Check sheet for the modelled part. Datum: model origin and axes. Units: mm. Face numbers are marked on the shaded views. Coordinates: 2 decimals unless noted, no trailing zeros. Loops run counter-clockwise (first coordinate to the right, second up) from the corner with the lowest first, then second, coordinate; pieces in that order, holes last. Notation, with made-up numbers: (54, 77) -> (111, 77) arc R26 cw to (111, 101) -> close; hole circle Ø7 at (-3.5, 83.25). An arc over 180 degrees is marked (long way). Use CSV: the item, a comma, the result in double quotes.
```python
from build123d import *

# Parameters (mm, degrees)
CROQUIS1_R              = 22.05
CROQUIS1_R_2            = 20.05
SALIENTE_EXTRUIR1_DEPTH = 16
CROQUIS1_4_R            = 17.95
CROQUIS1_4_R_2          = 16.2
SALIENTE_EXTRUIR2_DEPTH = 12.5
SALIENTE_EXTRUIR4_START = -5
CROQUIS1_6_R            = 22.05
CROQUIS1_6_R_2          = 20.05
CROQUIS1_6_R_3          = 17.95
CROQUIS1_6_R_4          = 16.2
SALIENTE_EXTRUIR4_DEPTH = 5
CORTAR_EXTRUIR1_REACH   = 39.595
CROQUIS4_R              = 11.05
CROQUIS4_R_2            = 1.25
CROQUIS5_R              = 2.5
CROQUIS5_R_2            = 1.25
CORTAR_EXTRUIR2_DEPTH   = 3
REDONDEO1_R             = 1
REDONDEO3_R             = 1
REDONDEO4_R             = 1


with BuildPart() as part:
    # Croquis1 → Saliente-Extruir1 (new body)
    with BuildSketch(Plane(origin=(0, 0, 0), x_dir=(1, 0, 0), z_dir=(0, 1, 0))):
        with Locations(Location((0, 0, 0), (0, 0, 270))):
            Circle(CROQUIS1_R)
        with Locations(Location((0, 0, 0), (0, 0, 270))):
            Circle(CROQUIS1_R_2, mode=Mode.SUBTRACT)
    extrude(amount=SALIENTE_EXTRUIR1_DEPTH)



with BuildPart() as body_2:
    # Croquis1_4 → Saliente-Extruir2 (new body)
    with BuildSketch(Plane(origin=(0, 0, 0), x_dir=(1, 0, 0), z_dir=(0, 1, 0))):
        with Locations(Location((0, 0, 0), (0, 0, 270))):
            Circle(CROQUIS1_4_R)
        with Locations(Location((0, 0, 0), (0, 0, 270))):
            Circle(CROQUIS1_4_R_2, mode=Mode.SUBTRACT)
    extrude(amount=SALIENTE_EXTRUIR2_DEPTH)


with BuildPart() as part_1:
    add(part.part)

    add(body_2.part)  # Saliente-Extruir4 merges body 2
    # Croquis1_6 → Saliente-Extruir4 (add)
    # profile 1 of 4: a face of its own
    with BuildSketch(Plane(origin=(0, 0, 0), x_dir=(1, 0, 0), z_dir=(0, 1, 0)).offset(SALIENTE_EXTRUIR4_START)):
        with Locations(Location((0, 0, 0), (0, 0, 270))):
            Circle(CROQUIS1_6_R)
        with Locations(Location((0, 0, 0), (0, 0, 270))):
            Circle(CROQUIS1_6_R_2, mode=Mode.SUBTRACT)
    # profile 2 of 4: a face of its own
    with BuildSketch(Plane(origin=(0, 0, 0), x_dir=(1, 0, 0), z_dir=(0, 1, 0)).offset(SALIENTE_EXTRUIR4_START)):
        with Locations(Location((0, 0, 0), (0, 0, 270))):
            Circle(CROQUIS1_6_R_2)
        with Locations(Location((0, 0, 0), (0, 0, 270))):
            Circle(CROQUIS1_6_R_3, mode=Mode.SUBTRACT)
    # profile 3 of 4: a face of its own
    with BuildSketch(Plane(origin=(0, 0, 0), x_dir=(1, 0, 0), z_dir=(0, 1, 0)).offset(SALIENTE_EXTRUIR4_START)):
        with Locations(Location((0, 0, 0), (0, 0, 270))):
            Circle(CROQUIS1_6_R_3)
        with Locations(Location((0, 0, 0), (0, 0, 270))):
            Circle(CROQUIS1_6_R_4, mode=Mode.SUBTRACT)
    # profile 4 of 4: a face of its own
    with BuildSketch(Plane(origin=(0, 0, 0), x_dir=(1, 0, 0), z_dir=(0, 1, 0)).offset(SALIENTE_EXTRUIR4_START)):
        with Locations(Location((0, 0, 0), (0, 0, 270))):
            Circle(CROQUIS1_6_R_4)
    extrude(amount=SALIENTE_EXTRUIR4_DEPTH)

    # Croquis4 → Cortar-Extruir1 (cut, up to next)
    with BuildSketch(Plane.XZ.offset(5), mode=Mode.PRIVATE) as cortar_extruir1_sk1:
        with Locations(Location((0, 0, 0), (0, 0, 270))):
            Circle(CROQUIS4_R)
    cortar_extruir1_tool1 = extrude(cortar_extruir1_sk1.sketch, amount=-CORTAR_EXTRUIR1_REACH, mode=Mode.PRIVATE) & part_1.part
    # Croquis4 → Cortar-Extruir1 (cut, up to next)
    with BuildSketch(Plane.XZ.offset(5), mode=Mode.PRIVATE) as cortar_extruir1_sk2:
        with Locations(Location((9.1, 12.1, 0), (0, 0, 270))):
            Circle(CROQUIS4_R_2)
    cortar_extruir1_tool2 = extrude(cortar_extruir1_sk2.sketch, amount=-CORTAR_EXTRUIR1_REACH, mode=Mode.PRIVATE) & part_1.part
    # Croquis4 → Cortar-Extruir1 (cut, up to next)
    with BuildSketch(Plane.XZ.offset(5), mode=Mode.PRIVATE) as cortar_extruir1_sk3:
        with Locations(Location((-9.1, -12.1, 0), (0, 0, 270))):
            Circle(CROQUIS4_R_2)
    cortar_extruir1_tool3 = extrude(cortar_extruir1_sk3.sketch, amount=-CORTAR_EXTRUIR1_REACH, mode=Mode.PRIVATE) & part_1.part
    add(cortar_extruir1_tool1.solids().sort_by_distance((0, -5, 0))[0], mode=Mode.SUBTRACT)
    add(cortar_extruir1_tool2.solids().sort_by_distance((9.1, -5, 12.1))[0], mode=Mode.SUBTRACT)
    add(cortar_extruir1_tool3.solids().sort_by_distance((-9.1, -5, -12.1))[0], mode=Mode.SUBTRACT)

    # Croquis5 → Cortar-Extruir2 (cut)
    # profile 1 of 2: a face of its own
    with BuildSketch(Plane.XZ.offset(5)):
        with Locations(Location((9.1, 12.1, 0), (0, 0, 270))):
            Circle(CROQUIS5_R)
        with Locations(Location((9.1, 12.1, 0), (0, 0, 270))):
            Circle(CROQUIS5_R_2, mode=Mode.SUBTRACT)
    # profile 2 of 2: a face of its own
    with BuildSketch(Plane.XZ.offset(5)):
        with Locations(Location((-9.1, -12.1, 0), (0, 0, 270))):
            Circle(CROQUIS5_R)
        with Locations(Location((-9.1, -12.1, 0), (0, 0, 270))):
            Circle(CROQUIS5_R_2, mode=Mode.SUBTRACT)
    extrude(amount=-CORTAR_EXTRUIR2_DEPTH, mode=Mode.SUBTRACT)

    # Redondeo1
    redondeo1_edges = [part_1.edges().sort_by_distance(p)[0] for p in [
        (0, -5, 11.05),
    ]]
    fillet(redondeo1_edges, radius=REDONDEO1_R)

    # Redondeo3
    redondeo3_edges = [part_1.edges().sort_by_distance(p)[0] for p in [
        (0, -5, -22.05),
    ]]
    fillet(redondeo3_edges, radius=REDONDEO3_R)

    # Redondeo4
    redondeo4_edges = [part_1.edges().sort_by_distance(p)[0] for p in [
        (0, 12.5, -17.95),
        (0, 16, -20.05),
    ]]
    fillet(redondeo4_edges, radius=REDONDEO4_R)


solid = part_1.part
```
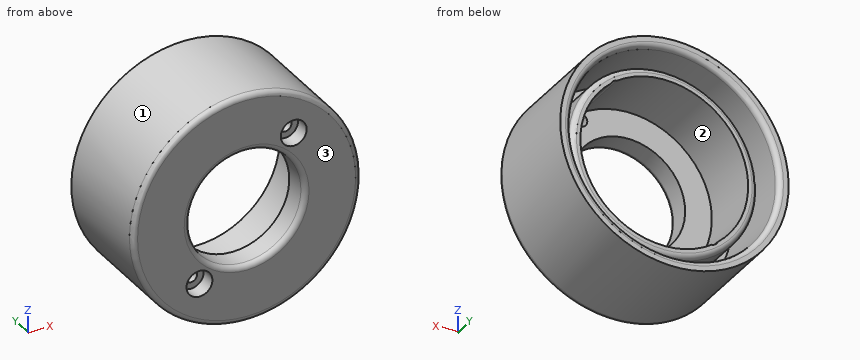
1) Cross-section at C-C on z = 0. Record the boundary of the cut face in (x, y), and give its area (3 significant figures).
Answer below:
outline,"(-22.05, -4) arc R1 ccw to (-21.05, -5) -> (-12.05, -5) arc R1 ccw to (-11.05, -4) -> (-11.05, 0) -> (-16.2, 0) -> (-16.2, 12.5) -> (-16.95, 12.5) arc R1 ccw to (-17.95, 11.5) -> (-17.95, 0) -> (-20.05, 0) -> (-20.05, 15) arc R1 ccw to (-21.05, 16) -> (-22.05, 16) -> close; (11.05, -4) arc R1 ccw to (12.05, -5) -> (21.05, -5) arc R1 ccw to (22.05, -4) -> (22.05, 16) -> (21.05, 16) arc R1 ccw to (20.05, 15) -> (20.05, 0) -> (17.95, 0) -> (17.95, 11.5) arc R1 ccw to (16.95, 12.5) -> (16.2, 12.5) -> (16.2, 0) -> (11.05, 0) -> close"
area,"216 mm²"
2) Thickness scan on line 1 along X through (y, z) = (8.5, 0); line 2 along X through (y, z) = (-0.9, 0); line 3 along Z through (x, y) = (-0.5, 6). Record the ranges inside material, lowest first. Write a range as from..to.
Answer below:
line 1,"x = -22.05..-20.05, -17.95..-16.2, 16.2..17.95, 20.05..22.05"
line 2,"x = -22.05..-11.05, 11.05..22.05"
line 3,"z = -22.04..-20.04, -17.94..-16.19, 16.19..17.94, 20.04..22.04"
3) Cross-section at A-A on y = 8.25. Record the boundary of the cut face in (x, z), and give its area (3 significant figures).
Answer below:
outline,"circle Ø44.1 at (0, 0); circle Ø35.9 at (0, 0); hole circle Ø40.1 at (0, 0); hole (-10.28, -12.52) arc R1.25 ccw to (-9.18, -13.35) arc R16.2 ccw to (10.28, 12.52) arc R1.25 ccw to (9.18, 13.35) arc R16.2 ccw to start"
area,"452 mm²"
4) Draft check along Z on the marked faces 1, 2 and 3. Enter one of: released by +Z, released by -Z, zero draft, split by the parting line, or undercut.
Answer below:
face 1,"split by the parting line"
face 2,"undercut"
face 3,"zero draft"
5) Cross-section at B-B on x = 0. Record the boundary of the cut face in (y, z).
Answer below:
outline,"(-5, -21.05) arc R1 ccw to (-4, -22.05) -> (16, -22.05) -> (16, -21.05) arc R1 ccw to (15, -20.05) -> (0, -20.05) -> (0, -17.95) -> (11.5, -17.95) arc R1 ccw to (12.5, -16.95) -> (12.5, -16.2) -> (0, -16.2) -> (0, -11.05) -> (-4, -11.05) arc R1 ccw to (-5, -12.05) -> close; (-5, 12.05) arc R1 ccw to (-4, 11.05) -> (0, 11.05) -> (0, 16.2) -> (12.5, 16.2) -> (12.5, 16.95) arc R1 ccw to (11.5, 17.95) -> (0, 17.95) -> (0, 20.05) -> (15, 20.05) arc R1 ccw to (16, 21.05) -> (16, 22.05) -> (-4, 22.05) arc R1 ccw to (-5, 21.05) -> close"
6) Go/stop test with flat-tipped pins: pin 1 Ø1 at (x, y) = (-10, 5.5) entering from -Z; pin 2 Ø5 at (x, z) = (-4.5, 8) entering from +Y; pin 3 Ø1 at (y, z) = (4.5, 0) entering from +X; pin 4 Ø6 at (x, z) = (9.1, 12.1) entering from -Y. Record where each tip stops, or that it passes through.
Answer below:
pin 1,"stops at z = -19.9"
pin 2,"stops at y = 0"
pin 3,"stops at x = 22.05"
pin 4,"stops at y = -5"
